from build123d import *

# Parameters (mm, degrees)
SKETCH045_R  = 23.7
PAD019_DEPTH = 2
SKETCH046_R  = 5
PAD020_DEPTH = 3
SKETCH047_R  = 3
PAD021_DEPTH = 4
SKETCH048_R  = 5
PAD022_DEPTH = 3
FILLET_R     = 1.999
FILLET001_R  = 1.9999
FILLET002_R  = 1


with BuildPart() as part:
    # Sketch045 (on Face1 of CopyPocket022) → Pad019 (new body)
    with BuildSketch(Plane.XY.offset(60)):
        Circle(SKETCH045_R)
    extrude(amount=PAD019_DEPTH)

    # Sketch046 (on Face3 of Pad019) → Pad020 (join)
    with BuildSketch(Plane.XY.offset(62)):
        Circle(SKETCH046_R)
    extrude(amount=PAD020_DEPTH)

    # Sketch047 (on Face5 of Pad020) → Pad021 (join)
    with BuildSketch(Plane.XY.offset(65)):
        Circle(SKETCH047_R)
    extrude(amount=PAD021_DEPTH)

    # Sketch048 (on Face7 of Pad021) → Pad022 (join)
    with BuildSketch(Plane.XY.offset(69)):
        Circle(SKETCH048_R)
    extrude(amount=PAD022_DEPTH)

    # Fillet
    fillet_edges = [part.edges().sort_by_distance(p)[0] for p in [
        (-3, 0, 65),
    ]]
    fillet(fillet_edges, radius=FILLET_R)

    # Fillet001
    fillet001_edges = [part.edges().sort_by_distance(p)[0] for p in [
        (-3, 0, 69),
    ]]
    fillet(fillet001_edges, radius=FILLET001_R)

    # Fillet002
    fillet002_edges = [part.edges().sort_by_distance(p)[0] for p in [
        (-5, 0, 72),
    ]]
    fillet(fillet002_edges, radius=FILLET002_R)


solid = part.part
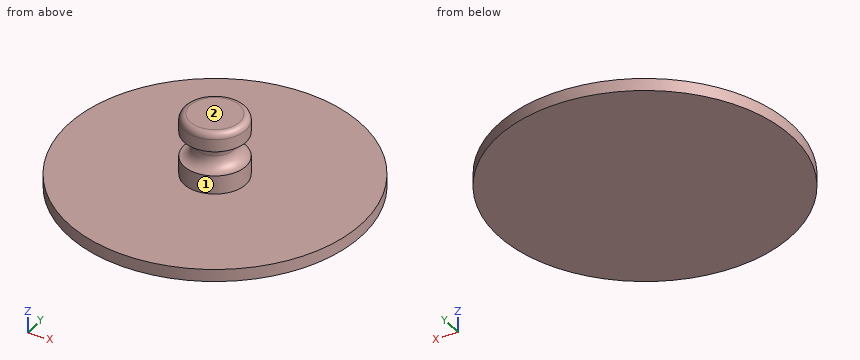
Verification items for the finished model (mm, model axes). Face numbers are marked on the shaded views. A direction names the side the tool comes from. Coordinates: 2 decimals unless noted, no trailing zeros. Order: outer loops, then holes, each group sorted by start corner. A loop starts at its lowest first (then second) coordinate and runs counter-clockwise, first axis right, second up. Notation, with made-up numbers: M -40,58.5 L 9,58.5 A14 ccw 9,72.5 Z; hole C 14,88.5 d1. An arc over 180 degrees is marked long. One line per item, written item: value. Start each with the question number.
Item 1: Access from +Z, -Z, +X, -X, +Y, -Y to the whole of each face (thin tool, end or side, straight path). Record for the marked faces 1 and 2.
Item 2: Scan lines: probe 1 along Z at (x, y) = (-14.5, -1.5); probe 2 along Y at (x, z) = (-2.5, 65.75); probe 3 along X at (y, z) = (1.5, 61.25). Record each from-to range of solid material in increasing order.
Item 3: Sectioned sample at C-C (y = -9). Enter the section's corners in (x, z).
Item 4: Gauge pin test, flat ends, axial feed: pin 1 (1 mm diameter, centred on x = -2, y = -9, fed in from +Z); pin 2 (6 mm diameter, centred on y = 5, z = 66.5, fed in from -X). Record the tip position at first contact, or that the pin passes through.
Item 5: Sectioned sample at D-D (x = 14.5). Enter the section's corners in (y, z), then the cut area to 3 significant figures.
Conclusion:
1. face 1: +Z
1. face 2: +Z, +X, -X, +Y, -Y
2. probe 1: z = 60 to 62
2. probe 2: y = -2.36 to 2.36
2. probe 3: x = -23.65 to 23.65
3. outline: M -21.92,60 L 21.92,60 L 21.92,62 L -21.92,62 Z
4. pin 1: stops at z = 62
4. pin 2: stops at x = -4.39
5. outline: M -18.75,60 L 18.75,60 L 18.75,62 L -18.75,62 Z
5. area: 75.0 mm^2
